Build history of the part. All positions in model axes, mm. Coordinates: 2 decimals unless noted, no trailing zeros. Order: outer loops, then holes, each group sorted by start corner. A loop starts at its lowest first (then second) coordinate and runs counter-clockwise, first axis right, second up. Notation, with made-up numbers: M 33.5,76 L 89.5,76 A19 cw 89.5,105 Z; hole C -9,16.25 d10. An arc over 180 degrees is marked long. Write item = value, one per line. Start each with the question number.
Q1. Drill centre lines: probe 1 along Y at (x, z) = (149, 1.25); probe 2 along X at (y, z) = (-120.5, 3.3); probe 3 along Y at (x, z) = (93, 0.4). Where is each one in solid material? Low to high.
Q2. Pin check, flat tips, straight feed: P1, Ø19, axis at x = -213.72, y = 69.5, coming from the +Z side; P2, Ø7, axis at x = -157.47, y = -120.5, coming from the -Z side. Stop position of each tip, or through.
Q3. Band-saw the part on B-B on x = -116. Write the cut outline in (y, z).
Q4. Band-saw the part on D-D on y = 24. Write the cut outline in (x, z).
Q5. Pull direction Y, two halves, no side cores. Call faces 1 (the face through (11, 117, 0)), 2 (the face through (98.524, -120.764, 2.535)): released by +Y, released by -Y, zero draft, split by the parting line, or undercut.
Q6. Band-saw the part on C-C on z = 3.75. State how many separate pieces and enclosed holes the cut face has, plus the area to 3 significant figures.
Q7. Band-saw the part on A-A on y = -55.5. Write the cut outline in (x, z).
```python
from build123d import *

# Parameters (mm, degrees)
SKETCH1_W           = 402.5
SKETCH1_H           = 295
SKETCH1_W_2         = 322.5
SKETCH1_H_2         = 215
BOSS_EXTRUDE1_DEPTH = 5
SKETCH2_R           = 6
CUT_EXTRUDE1_DEPTH  = 5


with BuildPart() as part:
    # Sketch1 → Boss-Extrude1 (new body)
    with BuildSketch(Plane.XY):
        with Locations((-32.469887955, 7)):
            Rectangle(SKETCH1_W, SKETCH1_H)
        with Locations((-32.469887955, 7)):
            Rectangle(SKETCH1_W_2, SKETCH1_H_2, mode=Mode.SUBTRACT)
    extrude(amount=BOSS_EXTRUDE1_DEPTH)

    # Sketch2 → Cut-Extrude1 (cut)
    with BuildSketch(Plane.XY.offset(5)):
        with Locations((-213.719887955, 69.5)):
            Circle(SKETCH2_R)
        with Locations((-213.719887955, -55.5)):
            Circle(SKETCH2_R)
        with Locations(Location((-157.469887955, -120.5, 0), (0, 0, 180))):
            Circle(SKETCH2_R)
        with Locations(Location((-32.469887955, -120.5, 0), (0, 0, 180))):
            Circle(SKETCH2_R)
        with Locations(Location((92.530112045, -120.5, 0), (0, 0, 180))):
            Circle(SKETCH2_R)
        with Locations((92.530112045, 134.5)):
            Circle(SKETCH2_R)
        with Locations((-32.469887955, 134.5)):
            Circle(SKETCH2_R)
        with Locations((-157.469887955, 134.5)):
            Circle(SKETCH2_R)
        with Locations(Location((148.780112045, -55.5, 0), (0, 0, 180))):
            Circle(SKETCH2_R)
        with Locations(Location((148.780112045, 69.5, 0), (0, 0, 180))):
            Circle(SKETCH2_R)
    extrude(amount=-CUT_EXTRUDE1_DEPTH, mode=Mode.SUBTRACT)


solid = part.part
```
Recorded:
q1.probe_1 = -140.5 to -61.5, -49.5 to 63.5, 75.5 to 154.5
q1.probe_2 = -233.72 to -163.47, -151.47 to -38.47, -26.47 to 86.53, 98.53 to 168.78
q1.probe_3 = -140.5 to -126.48, -114.52 to -100.5, 114.5 to 128.52, 140.48 to 154.5
q2.P1 = 5
q2.P2 = through
q3.outline = M -140.5,0 L -100.5,0 L -100.5,5 L -140.5,5 Z; M 114.5,0 L 154.5,0 L 154.5,5 L 114.5,5 Z
q4.outline = M -233.72,0 L -193.72,0 L -193.72,5 L -233.72,5 Z; M 128.78,0 L 168.78,0 L 168.78,5 L 128.78,5 Z
q5.face_1 = zero draft
q5.face_2 = undercut
q6.separate_pieces = 1
q6.enclosed_holes = 11
q6.area = 48,300 mm2
q7.outline = M -233.72,0 L -219.72,0 L -219.72,5 L -233.72,5 Z; M -207.72,0 L -193.72,0 L -193.72,5 L -207.72,5 Z; M 128.78,0 L 142.78,0 L 142.78,5 L 128.78,5 Z; M 154.78,0 L 168.78,0 L 168.78,5 L 154.78,5 Z
